Answer from the drawing. Dimensions are ordinates in mm from the lowest x, y and z of the part. A direction names the side the tool comes from. Round coordinates to 2 decimals unless told otherwise and drop trailing zeros. Loops run counter-clockwise (first coordinate to the right, second up) from the corner with the lowest first, then second, coordinate; pieces in that order, holes last.
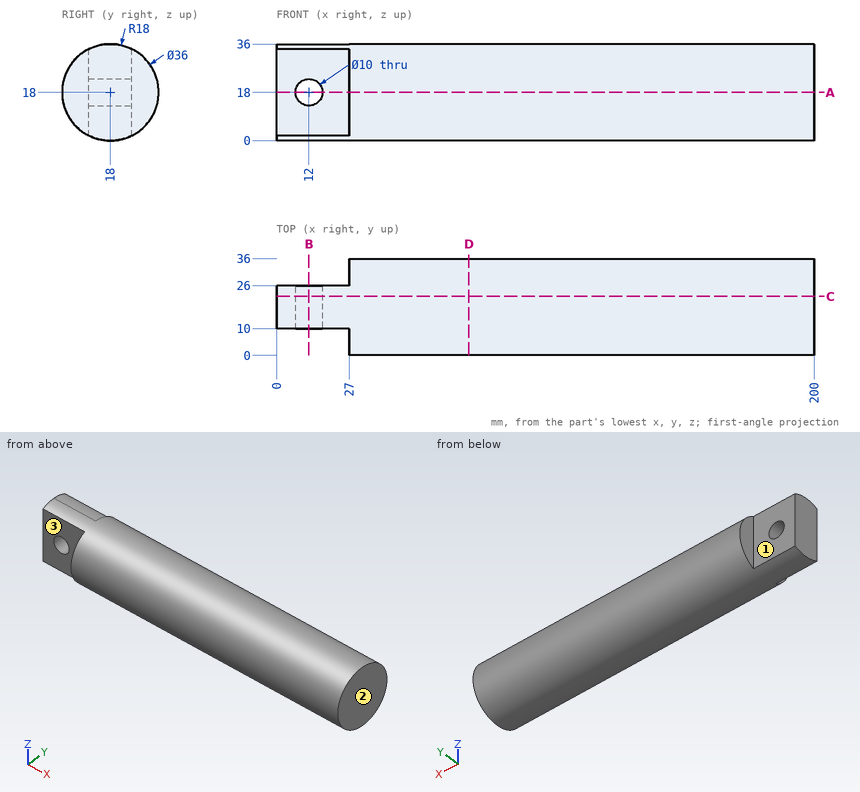
1. Find section C-C (y = 22). Write down the section's boundary in (x, z), then the cut area to 3 significant figures.
Answer key:
outline: (0, 0.45) - (200, 0.45) - (200, 35.55) - (0, 35.55) - close; hole circle Ø10 at (12, 18)
area: 6,940 mm2
2. Find section D-D (x = 71.5). Write down the section's boundary in (y, z), then the cut area to 3 significant figures.
Answer key:
outline: circle Ø36 at (18, 18)
area: 1,020 mm2
3. Find section B-B (x = 12). Write down the section's boundary in (y, z), then the cut area to 3 significant figures.
Answer key:
outline: (10, 1.88) arc R18 ccw to (26, 1.88) - (26, 13) - (10, 13) - close; (10, 23) - (26, 23) - (26, 34.12) arc R18 ccw to (10, 34.12) - close
area: 396 mm2
4. Which of the six approach directions +Z, -Z, +X, -X, +Y, -Y give full straight-line access (tool end or side, diameter ignored) to the marked faces 1, 2 and 3?
Answer key:
face 1: +Z, -Z, -X, +Y
face 2: +Z, -Z, +X, +Y, -Y
face 3: +Z, -Z, -X, -Y
5. Consider probe 1 along X at (y, z) = (16, 18); probe 2 along Z at (x, y) = (12, 19); probe 3 along X at (y, z) = (4.5, 28). Determine where each line is inside the solid, lowest interval first.
Answer key:
probe 1: x = 0 to 7, 17 to 200
probe 2: z = 0.03 to 13, 23 to 35.97
probe 3: x = 27 to 200
6. Find section A-A (z = 18). Write down the section's boundary in (x, y).
Answer key:
outline: (0, 10) - (7, 10) - (7, 26) - (0, 26) - close; (17, 10) - (27, 10) - (27, 0) - (200, 0) - (200, 36) - (27, 36) - (27, 26) - (17, 26) - close
7. Given pin 1 (10 mm diameter, centred on x = 87.5, z = 12.5, fed in from +Y); pin 2 (11.5 mm diameter, centred on x = 12, z = 18, fed in from -Y); pin 3 (8 mm diameter, centred on x = 8.5, z = 22.5, fed in from +Y), each flat-ended and moving along its own axis, determine where each tip first touches the part or whether it passes through.
Answer key:
pin 1: stops at y = 35.99
pin 2: stops at y = 10
pin 3: stops at y = 26
